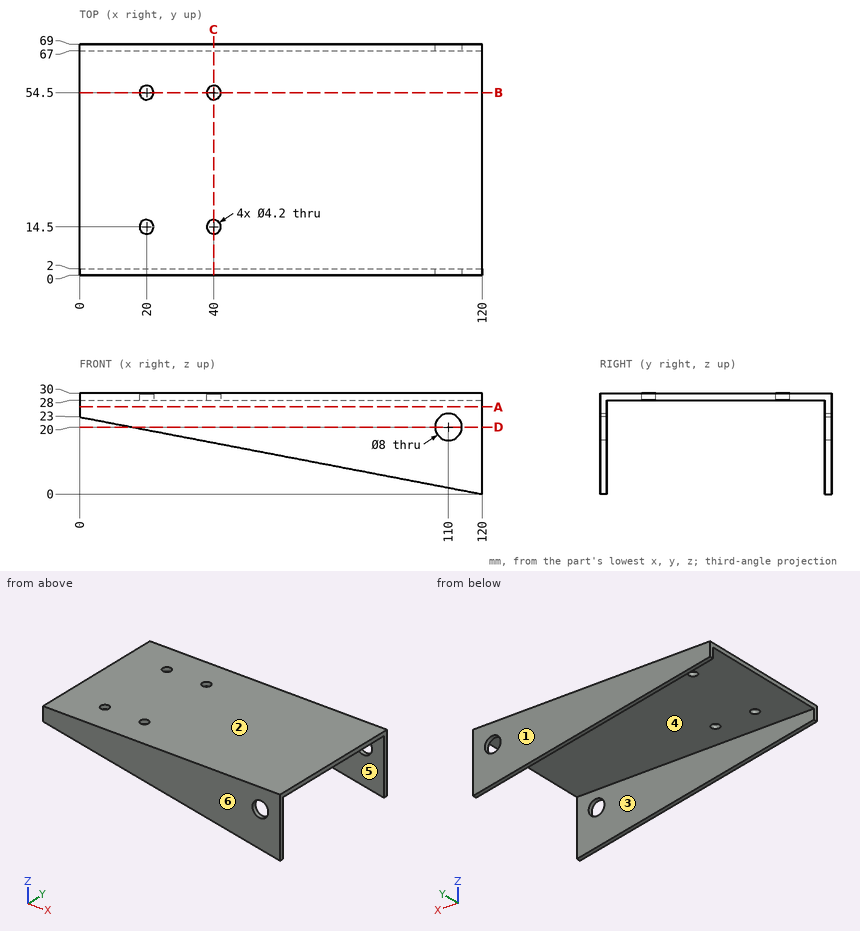
Print and shaded views of the part. All mm, measured from the part's lowest x, y and z. A direction names the side the tool comes from. Coordinates: 2 decimals unless noted, no trailing zeros. Order: outer loops, then holes, each group sorted by start corner. A loop starts at its lowest first (then second) coordinate and runs counter-clockwise, first axis right, second up.
(1) Tool access for the marked faces 5 and 6: list every direction of +Z, -Z, +X, -X, +Y, -Y with a clear straight run to the whole face (end or side of a thin tool).
Check sheet entries:
face 5: -Z, +X, -X
face 6: +Z, -Z, +X, -X, -Y
(2) Slice it at B-B, the plane y = 54.5. Write the cut outline in (x, z), and give its area (3 significant figures).
Check sheet entries:
outline: (0, 28) - (17.9, 28) - (17.9, 30) - (0, 30) - close; (22.1, 28) - (37.9, 28) - (37.9, 30) - (22.1, 30) - close; (42.1, 28) - (120, 28) - (120, 30) - (42.1, 30) - close
area: 223 mm2
(3) Slice it at C-C, the plane x = 40. Write the cut outline in (y, z), and give its area (3 significant figures).
Check sheet entries:
outline: (0, 15.33) - (2, 15.33) - (2, 28) - (12.4, 28) - (12.4, 30) - (0, 30) - close; (16.6, 28) - (52.4, 28) - (52.4, 30) - (16.6, 30) - close; (56.6, 28) - (67, 28) - (67, 15.33) - (69, 15.33) - (69, 30) - (56.6, 30) - close
area: 172 mm2
(4) Pin check, flat tips, straight feed: pin 1 Ø5 at (x, y) = (20, 14.5) entering from -Z; pin 2 Ø3.5 at (x, y) = (40, 14.5) entering from +Z. Stop position of each tip, or through.
Check sheet entries:
pin 1: stops at z = 28
pin 2: passes through
(5) Slice it at D-D, the plane z = 20. Write the cut outline in (x, y), and give its area (3 significant figures).
Check sheet entries:
outline: (15.65, 0) - (106, 0) - (106, 2) - (15.65, 2) - close; (15.65, 67) - (106, 67) - (106, 69) - (15.65, 69) - close; (114, 0) - (120, 0) - (120, 2) - (114, 2) - close; (114, 67) - (120, 67) - (120, 69) - (114, 69) - close
area: 385 mm2
(6) Pull direction Y, two halves, no side cores. Call the marked faces 1, 2, 3 and 4: pulls with the +Y half, pulls with the -Y half, needs draft (parallel to the pull), parting line crosses it, or undercut.
Check sheet entries:
face 1: pulls with the +Y half
face 2: needs draft
face 3: undercut
face 4: undercut
(7) Slice it at A-A, the plane z = 26. Write the cut outline in (x, y), and give its area (3 significant figures).
Check sheet entries:
outline: (0, 0) - (120, 0) - (120, 2) - (0, 2) - close; (0, 67) - (120, 67) - (120, 69) - (0, 69) - close
area: 480 mm2
(8) Probe L1, parallel to Y at x = 20, z = 29.1; L2, parallel to Y at x = 100.5, z = 16.25; L3, parallel to Z at x = 89, y = 46. List the from-to ranges inside material, lowest first.
Check sheet entries:
L1: y = 0 to 12.4, 16.6 to 52.4, 56.6 to 69
L2: y = 0 to 2, 67 to 69
L3: z = 28 to 30
